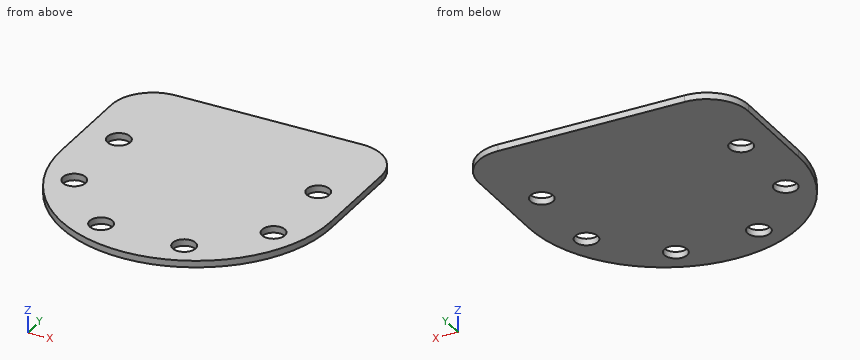
```python
from build123d import *

# Parameters (mm, degrees)
BOSS_EXTRUDE1_DEPTH  = 1.6002
M5_CLEARANCE_HOLE1_D = 5.5
FILLET1_R            = 10


with BuildPart() as part:
    # Sketch1 → Boss-Extrude1 (new body)
    with BuildSketch(Plane.XY):
        with BuildLine():
            Line((-32.5, 0), (-32.5, 32.5))
            Line((-32.5, 32.5), (32.5, 32.5))
            Line((32.5, 32.5), (32.5, 0))
            ThreePointArc((32.5, 0), (0, -32.5), (-32.5, 0))
        make_face()
    extrude(amount=BOSS_EXTRUDE1_DEPTH)

    # M5 Clearance Hole1 (through all)
    with Locations(Plane.XY.offset(1.6002)):
        with Locations((24, -10), (10, -24), (-10, -24), (-24, -10), (-24, 10), (24, 10)):
            Hole(M5_CLEARANCE_HOLE1_D / 2)

    # Fillet1
    fillet1_edges = [part.edges().sort_by_distance(p)[0] for p in [
        (-32.5, 32.5, 0.8001),
        (32.5, 32.5, 0.8001),
    ]]
    fillet(fillet1_edges, radius=FILLET1_R)


solid = part.part
```
Check sheet for the modelled part. Datum: model origin and axes. Units: mm. Round coordinates to 2 decimals unless told otherwise and drop trailing zeros. Loops run counter-clockwise (first coordinate to the right, second up) from the corner with the lowest first, then second, coordinate; pieces in that order, holes last. Notation, with made-up numbers: (35.25, -10.5) - (60.25, -10.5) arc R22 ccw to (60.25, 15.5) - close; hole circle Ø7 at (58, 15.5). An arc over 180 degrees is marked (long way). Write item = value, one per line. Start each with the question number.
Q1. Section check B-B (x = -24). Record the boundary of the cut face in (y, z).
Q2. Depth check by flat-ended pin: P1, Ø9, axis at x = -24, y = 10, coming from the -Z side. Enter the tip coordinate at first touch or a pass-through.
Q3. Section check D-D (x = 11). Record the boundary of the cut face in (y, z).
Q4. Thickness scan on L1, parallel to Y at x = 24, z = 1.15; L2, parallel to X at y = -10.5, z = 1.1; L3, parallel to X at y = -25, z = 1.25. Record the ranges inside material, lowest first.
Q5. Section check C-C (z = 0.75). Record the boundary of the cut face in (x, y).
Q6. Section check A-A (y = 10). Record the boundary of the cut face in (x, z).
Derived:
q1.outline = (-21.91, 0) - (-12.75, 0) - (-12.75, 1.6) - (-21.91, 1.6) - close; (-7.25, 0) - (7.25, 0) - (7.25, 1.6) - (-7.25, 1.6) - close; (12.75, 0) - (32.39, 0) - (32.39, 1.6) - (12.75, 1.6) - close
q2.P1 = 0
q3.outline = (-30.58, 0) - (-26.56, 0) - (-26.56, 1.6) - (-30.58, 1.6) - close; (-21.44, 0) - (32.5, 0) - (32.5, 1.6) - (-21.44, 1.6) - close
q4.L1 = -21.91 to -12.75, -7.25 to 7.25, 12.75 to 32.39
q4.L2 = -30.76 to -26.7, -21.3 to 21.3, 26.7 to 30.76
q4.L3 = -20.77 to -12.56, -7.44 to 7.44, 12.56 to 20.77
q5.outline = (-32.5, 0) arc R32.5 ccw to (32.5, 0) - (32.5, 22.5) arc R10 ccw to (22.5, 32.5) - (-22.5, 32.5) arc R10 ccw to (-32.5, 22.5) - close; hole circle Ø5.5 at (-24, -10); hole circle Ø5.5 at (-24, 10); hole circle Ø5.5 at (-10, -24); hole circle Ø5.5 at (10, -24); hole circle Ø5.5 at (24, -10); hole circle Ø5.5 at (24, 10)
q6.outline = (-32.5, 0) - (-26.75, 0) - (-26.75, 1.6) - (-32.5, 1.6) - close; (-21.25, 0) - (21.25, 0) - (21.25, 1.6) - (-21.25, 1.6) - close; (26.75, 0) - (32.5, 0) - (32.5, 1.6) - (26.75, 1.6) - close
